Here's how the part is built. I have some questions about the finished solid (model axes, mm). Coordinates: 2 decimals unless noted, no trailing zeros. Order: outer loops, then holes, each group sorted by start corner. A loop starts at its lowest first (then second) coordinate and runs counter-clockwise, first axis right, second up.
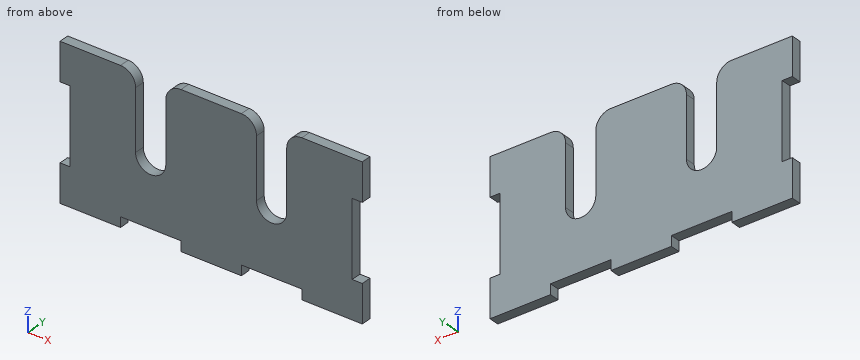
```python
from build123d import *

# Parameters (mm, degrees)
SKETCH1_W           = 90
SKETCH1_H           = 45
BOSS_EXTRUDE1_DEPTH = 3
CUT_EXTRUDE1_DEPTH  = 3
FILLET1_R           = 4.5
SKETCH4_W           = 3
SKETCH4_H           = 22.5
SKETCH4_W_2         = 18
SKETCH4_H_2         = 3
CUT_EXTRUDE4_DEPTH  = 3


with BuildPart() as part:
    # Sketch1 → Boss-Extrude1 (new body)
    with BuildSketch(Plane(origin=(0, 0, 0), x_dir=(1, 0, 0), z_dir=(0, 1, 0))):
        Rectangle(SKETCH1_W, SKETCH1_H)
    extrude(amount=BOSS_EXTRUDE1_DEPTH)

    # Sketch2 → Cut-Extrude1 (cut)
    with BuildSketch(Plane(origin=(0, 3, 0), x_dir=(1, 0, 0), z_dir=(0, 1, 0))):
        with BuildLine():
            Line((-22.5, -22.5), (-13.5, -22.5))
            Line((-13.5, -22.5), (-13.5, 0))
            ThreePointArc((-13.5, 0), (-18, 4.5), (-22.5, 0))
            Line((-22.5, 0), (-22.5, -22.5))
        make_face()
        with BuildLine():
            Line((13.5, -22.5), (22.5, -22.5))
            Line((22.5, -22.5), (22.5, 0))
            ThreePointArc((22.5, 0), (18, 4.5), (13.5, 0))
            Line((13.5, 0), (13.5, -22.5))
        make_face()
    extrude(amount=-CUT_EXTRUDE1_DEPTH, mode=Mode.SUBTRACT)

    # Fillet1
    fillet1_edges = [part.edges().sort_by_distance(p)[0] for p in [
        (-22.5, 1.5, 22.5),
        (-13.5, 1.5, 22.5),
        (13.5, 1.5, 22.5),
        (22.5, 1.5, 22.5),
    ]]
    fillet(fillet1_edges, radius=FILLET1_R)

    # Sketch4 → Cut-Extrude4 (cut)
    with BuildSketch(Plane(origin=(0, 3, 0), x_dir=(1, 0, 0), z_dir=(0, 1, 0))):
        with Locations((-43.5, 0)):
            Rectangle(SKETCH4_W, SKETCH4_H)
        with Locations((-18, 21)):
            Rectangle(SKETCH4_W_2, SKETCH4_H_2)
        with Locations((18, 21)):
            Rectangle(SKETCH4_W_2, SKETCH4_H_2)
        with Locations((43.5, 0)):
            Rectangle(SKETCH4_W, SKETCH4_H)
    extrude(amount=-CUT_EXTRUDE4_DEPTH, mode=Mode.SUBTRACT)


solid = part.part
```
Q1. I need wall thicknesses on L1, parallel to X at y = 1.25, z = 3.5; L2, parallel to X at y = 2.55, z = 15.5; L3, parallel to X at y = 0.35, z = -6. Which ranges of each line are inside material? Lowest first, please.
Q2. Will these pins go through, and if not, where does the flat tip stop? pin 1 (3 mm diameter, centred on x = 12, z = -1, fed in from -Y); pin 2 (1.5 mm diameter, centred on y = 1.5, z = 7, fed in from +X).
Q3. If we section it at D-D on x = -18: Write out the boundary of the cut face in (y, z), then the cut area to 3 significant figures.
Q4. If we section it at C-C on z = 14: Write out the boundary of the cut face in (x, y).
Q5. If we section it at A-A on z = 7.5: Write out the boundary of the cut face in (x, y), then the cut area to 3 significant figures.
Reply:
1. L1: x = -42 to -22.5, -13.5 to 13.5, 22.5 to 42
1. L2: x = -45 to -22.5, -13.5 to 13.5, 22.5 to 45
1. L3: x = -42 to 42
2. pin 1: stops at y = 0
2. pin 2: stops at x = 42
3. outline: (0, -19.5) - (3, -19.5) - (3, -4.5) - (0, -4.5) - close
3. area: 45.0 mm2
4. outline: (-45, 0) - (-22.5, 0) - (-22.5, 3) - (-45, 3) - close; (-13.5, 0) - (13.5, 0) - (13.5, 3) - (-13.5, 3) - close; (22.5, 0) - (45, 0) - (45, 3) - (22.5, 3) - close
5. outline: (-42, 0) - (-22.5, 0) - (-22.5, 3) - (-42, 3) - close; (-13.5, 0) - (13.5, 0) - (13.5, 3) - (-13.5, 3) - close; (22.5, 0) - (42, 0) - (42, 3) - (22.5, 3) - close
5. area: 198 mm2
